Verification items for the finished model (mm, model axes). Give positions to 0.01 mm unless a question says otherwise; leave off trailing zeros. Write each loop counter-clockwise with the first axis right and the second up, starting at its lowest first coordinate (ties: lowest second). Pieces come first, ordered by that corner, then holes. Notation, with made-up numbers: (-14, 28) - (-3, 28) arc R17 cw to (-3, 40) - close; hole circle Ø5 at (63, -20.75). An arc over 180 degrees is marked (long way). Answer as a JSON object with one key per item and string values. Group by question number.
Item 1: Draft check along Y on faces 1 (the face through (30.5, 0, 1)), 2 (the face through (-29.9, 24.43, 0.76)), 3 (the face through (8.92, 22.74, 0.76)), 4 (the face through (29.9, -24.43, 0.76)). Enter one of: +Y half, -Y half, draft (parallel to the pull), parting line (faces both ways), or undercut.
Item 2: Scan lines: line 1 along Y through (x, z) = (-3.5, 0.45); line 2 along X through (y, z) = (22, 0.75); line 3 along Y through (x, z) = (8, 0.45). Record each from-to range of solid material in increasing order. Write a range as [from, to].
Item 3: Sectioned sample at B-B, the plane z = 0.6. Count the separate pieces of the cut face and the enclosed holes in it, and give its area (3 significant figures).
Item 4: Sectioned sample at A-A, the plane x = -27.5. Record the boundary of the cut face in (y, z), and give its area (3 significant figures).
Item 5: Sectioned sample at C-C, the plane y = -22. Record the boundary of the cut face in (x, z), and give its area (3 significant figures).
Autodesk Inventor part; units mm, degrees
ref_plane "YZ Plane" through (0, 0, 0) normal (1, 0, 0) x (0, 1, 0)
ref_plane "XZ Plane" through (0, 0, 0) normal (0, 1, 0) x (-1, 0, 0)
ref_plane "XY Plane" through (0, 0, 0) normal (0, 0, 1) x (1, 0, 0)
sketch "スケッチ1" plane through (0, 0, 0) normal (0, 0, 1) x (1, 0, 0)
  line L0 (-30.5, 25) -> (30.5, 25)
  line L1 (30.5, 25) -> (30.5, -25)
  line L2 (30.5, -25) -> (-30.5, -25)
  line L3 (-30.5, -25) -> (-30.5, 25)
  point P0 (0, 0)
  point P1 (-30.5, 0)
  point P2 (0, 25)
  point P3 (-27.5, 22)
  point P4 (7.5, 22)
  point P5 (7.5, -22)
  point P6 (-27.5, -22)
  point P7 (-3.5, -22)
  point P8 (-3.5, 22)
  point P9 (22.5, 22)
  point P10 (22.5, -22)
  dimension "d0" = 50
  dimension "d1" = 61
  dimension "d2" = 35
  dimension "d3" = 44
  dimension "d4" = 3
  dimension "d5" = 3
  dimension "d18" = 44
  dimension "d20" = 22
  dimension "d23" = 26
  dimension "d26" = 11
extrude "押し出し1" add sketch "スケッチ1" along normal blind 1.5
hole "穴1" at (-27.5, 22, 0) at (7.5, 22, 0) at (7.5, -22, 0) at (-27.5, -22, 0) at (-3.5, -22, 0) at (-3.5, 22, 0) at (22.5, 22, 0) at (22.5, -22, 0) direction (0, 0, 1) diameter 3.2 depth 8.8 tip angle 118
fillet "フィレット1" radius 2 4 edges at (30.5, 25, 0.75) (30.5, -25, 0.75) (-30.5, 25, 0.75) (-30.5, -25, 0.75)
properties part number "回収機構天井"
Geometry check:
{
 "1": {"face 1": "draft", "face 2": "+Y half", "face 3": "undercut", "face 4": "-Y half"},
 "2": {"line 1": "[-25, -23.6], [-20.4, 20.4], [23.6, 25]", "line 2": "[-30.5, -29.1], [-25.9, -5.1], [-1.9, 5.9], [9.1, 20.9], [24.1, 30.5]", "line 3": "[-25, -23.52], [-20.48, 20.48], [23.52, 25]"},
 "3": {"separate pieces": "1", "enclosed holes": "8", "area": "2,980 mm^2"},
 "4": {"outline": "(-25, 0) - (-23.6, 0) - (-23.6, 1.5) - (-25, 1.5) - close; (-20.4, 0) - (20.4, 0) - (20.4, 1.5) - (-20.4, 1.5) - close; (23.6, 0) - (25, 0) - (25, 1.5) - (23.6, 1.5) - close", "area": "65.4 mm^2"},
 "5": {"outline": "(-30.5, 0) - (-29.1, 0) - (-29.1, 1.5) - (-30.5, 1.5) - close; (-25.9, 0) - (-5.1, 0) - (-5.1, 1.5) - (-25.9, 1.5) - close; (-1.9, 0) - (5.9, 0) - (5.9, 1.5) - (-1.9, 1.5) - close; (9.1, 0) - (20.9, 0) - (20.9, 1.5) - (9.1, 1.5) - close; (24.1, 0) - (30.5, 0) - (30.5, 1.5) - (24.1, 1.5) - close", "area": "72.3 mm^2"}
}
